from build123d import *

# Parameters (mm, degrees)
F0_R      = 12.5
F0_R_2    = 10
F1_DEPTH  = 20
F4_R      = 12.5
F4_R_2    = 10
F5_DEPTH  = 50
F6_R      = 10
F7_DEPTH  = 25
F8_R      = 10
F9_DEPTH  = 25
F10_R     = 5
F11_DEPTH = 25
F13_R     = 5
F14_DEPTH = 15
F15_DEPTH = 10


with BuildPart() as f1:
    # F0 (on Front) → F1 (new body, symmetric)
    with BuildSketch(Plane.XZ):
        Circle(F0_R)
        Circle(F0_R_2, mode=Mode.SUBTRACT)
    extrude(amount=F1_DEPTH, both=True)

    # F4 (on line) → F5 (join)
    with BuildSketch(Plane(origin=(0, 0, 0), x_dir=(0.1952614984, 0.9807512158, 0), z_dir=(0.9807512158, -0.1952614984, 0))):
        Circle(F4_R)
        Circle(F4_R_2, mode=Mode.SUBTRACT)
    extrude(amount=-F5_DEPTH)

    # F6 (on Front) → F7 (cut, symmetric)
    with BuildSketch(Plane.XZ):
        Circle(F6_R)
    extrude(amount=F7_DEPTH, both=True, mode=Mode.SUBTRACT)

    # F8 (on line) → F9 (cut)
    with BuildSketch(Plane(origin=(0, 0, 0), x_dir=(0.1952614984, 0.9807512158, 0), z_dir=(0.9807512158, -0.1952614984, 0))):
        Circle(F8_R)
    extrude(amount=-F9_DEPTH, mode=Mode.SUBTRACT)

    # F10 (on Right) → F11 (cut)
    with BuildSketch(Plane.YZ):
        Circle(F10_R)
    extrude(amount=F11_DEPTH, mode=Mode.SUBTRACT)

    # F13 (on face) → F14 (cut, symmetric)
    with BuildSketch(Plane(origin=(0, 0, 0), x_dir=(-0.9807512158, 0.1952614984, 0), z_dir=(0.1952614984, 0.9807512158, 0))):
        with Locations((35, 0)):
            Circle(F13_R)
    extrude(amount=F14_DEPTH, both=True, mode=Mode.SUBTRACT)

    # F15 (add): a face of the model
    f15_faces = [f1.faces().sort_by_distance(p)[0] for p in [
        (-51.4092941538, -2.1495673612, 0),
    ]]
    extrude(f15_faces, amount=F15_DEPTH)


solid = f1.part
For this review, take the finished solid that the model builds, in its own axes (mm). A direction names the side the tool comes from. Round coordinates to 2 decimals unless told otherwise and drop trailing zeros. Write each loop counter-clockwise with the first axis right and the second up, starting at its lowest first coordinate (ties: lowest second). Pieces come first, ordered by that corner, then holes. Notation, with made-up numbers: (47, -36) - (99, -36) arc R15 ccw to (99, -30) - close; hole circle Ø8 at (37, 77). An arc over 180 degrees is marked (long way). Write item = value, one per line. Start each with the question number.
1. For faces 4 (the face through (5.38, 0.28, 8.43)), 5 (the face through (-0.1, 20, 10.2)), 6 (the face through (11, -5, 0)), 7 (the face through (11.923, -4.724, 3.755)), list the 3-axis set-ups (+Z, -Z, +X, -X, +Y, -Y) from which the entire face can be reached by the end or side of a thin tool; tool diameter is ignored.
2. For pin 1 Ø10 at (x, y) = (-18, -4) entering from -Z; pin 2 Ø6 at (x, y) = (-10.5, -7) entering from -Z; pin 3 Ø6 at (x, y) = (3.5, 0.5) entering from +Z; pin 4 Ø7.5 at (x, z) = (-0.5, -4.5) entering from +Y, all flat-tipped, find the tip position at first contact; note any pin that passes through.
3. Draft analysis for pull direction X (two halves, no side actions). For faces 1 (the face through (-0.1, -20, 10.2)), 2 (the face through (-31.45, -6.47, 0.55)), 3 (the face through (-58.856, 11.658, 10.244)), state which applies: released by +X, released by -X, zero draft, split by the parting line, or undercut.
4. Consider section A-A on z = 1.75. State the section outline as (x, y) points.
5. Wall thickness on L1, parallel to Y at x = 10.6, z = 0; L2, parallel to Z at x = 0, y = -7.5; L3, parallel to Y at x = -30.5, z = 7.5: over which ranges is each line inside the solid? List them lowest first.
6. Consider section B-B on z = -6. State the section outline as (x, y) points.
7. Consider section C-C on z = 6.5. State the section outline as (x, y) points, plus the area to 3 significant figures.
Evaluation:
q1.face_4 = +Y, -Y
q1.face_5 = +Z, -Z, +X, +Y
q1.face_6 = +X
q1.face_7 = none
q2.pin_1 = -12.26
q2.pin_2 = -11.01
q2.pin_3 = 12.49
q2.pin_4 = through
q3.face_1 = zero draft
q3.face_2 = undercut
q3.face_3 = released by -X
q4.outline = (-61.26, -0.42) - (-41.34, -4.39) - (-40.84, -1.91) - (-60.77, 2.06) - close; (-56.92, 21.37) - (-37, 17.4) - (-36.5, 19.89) - (-56.43, 23.85) - close; (-32.15, -6.22) - (-12.38, -10.16) - (-12.38, -20) - (-9.85, -20) - (-9.85, -8.08) - (-31.66, -3.74) - close; (-27.81, 15.58) - (-9.85, 12) - (-9.85, 20) - (-12.38, 20) - (-12.38, 15.08) - (-27.32, 18.06) - close; (9.85, -20) - (12.38, -20) - (12.38, -4.68) - (9.85, -4.68) - close; (9.85, 4.68) - (12.38, 4.68) - (12.38, 20) - (9.85, 20) - close
q5.L1 = -20 to -5, 5 to 20
q5.L2 = -12.5 to -10, 10 to 12.5
q5.L3 = -4.12 to -0.67, 12.82 to 16.27
q6.outline = (-60.99, 0.96) - (-10.97, -9) - (-10.97, -20) - (-8, -20) - (-8, -6.56) - (-60.41, 3.87) - close; (-57.28, 19.56) - (-8, 9.75) - (-8, 20) - (-10.97, 20) - (-10.97, 13.36) - (-56.7, 22.47) - close; (8, -20) - (10.97, -20) - (10.97, 20) - (8, 20) - close
q7.outline = (-60.93, 1.24) - (-10.68, -8.76) - (-10.68, -20) - (-7.6, -20) - (-7.6, -6.24) - (-60.33, 4.26) - close; (-57.36, 19.17) - (-7.6, 9.26) - (-7.6, 20) - (-10.68, 20) - (-10.68, 13.01) - (-56.76, 22.19) - close; (7.6, -20) - (10.68, -20) - (10.68, 20) - (7.6, 20) - close
q7.area = 501 mm2
